Part model, mm, in its own coordinate system. A direction names the side the tool comes from. Coordinates: 2 decimals unless noted, no trailing zeros. Order: outer loops, then holes, each group sorted by start corner. A loop starts at its lowest first (then second) coordinate and runs counter-clockwise, first axis right, second up.
1) Cut at C-C (z = -1.85). List the corners of the cut face in (x, y) (3 decimals).
2) Cut at B-B (y = 18). List the corners of the cut face in (x, z).
3) Wall check: L1, parallel to Y at x = 11, z = -2.2; L2, parallel to X at y = 13.25, z = -1.5; L3, parallel to Y at x = 5, z = -0.8 (3 decimals). Give the ranges that are in metal, low to high.
4) Cut at A-A (x = 5). List the corners of the cut face in (y, z) (3 decimals), and give its area (3 significant figures).
5) Mould opens along Y. For faces 6 (the cylindrical face through (14, 27, -1)), 7 (the cylindrical face through (11, 28, -1)), 8 (the cylindrical face through (8.6, 23.43, -1.48)), 9 (the flat face through (-10, 19, -3)) say: +Y half, -Y half, draft (parallel to the pull), parting line (faces both ways), or undercut.
6) Pin check, flat tips, straight feed: pin 1 Ø0.9 at (y, z) = (1, -1.5) entering from -X; pin 2 Ø1.5 at (y, z) = (17, -1) entering from +X; pin 3 Ø1.1 at (x, z) = (10.5, -1.5) entering from -Y. Stop position of each tip, or through.
7) Cut at D-D (x = -12). List the corners of the cut face in (y, z).
8) Tool access for faces 1 (the cylindrical face through (-19.85, 22.66, -1.48)), 2 (the flat face through (-32, 2.976, -1)), 3 (the flat face through (8, 14, -1)), 4 (the flat face through (-10, 19, 0)), 5 (the cylindrical face through (1.434, 20.389, -1.479)): list every direction of +Z, -Z, +X, -X, +Y, -Y with a clear straight run to the whole face (end or side of a thin tool).
Autodesk Inventor part; units mm, degrees
ref_plane "YZ Plane" through (0, 0, 0) normal (1, 0, 0) x (0, 1, 0)
ref_plane "XZ Plane" through (0, 0, 0) normal (0, 1, 0) x (-1, 0, 0)
ref_plane "XY Plane" through (0, 0, 0) normal (0, 0, 1) x (1, 0, 0)
sketch "Sketch1" plane through (0, 0, 0) normal (0, 0, 1) x (1, 0, 0)
  arc A0 (0, 18) -> (-18, 0.0024) centre (0, 0) ccw
  line L0 (0, 0) -> (0, -6.19)
  line L1 (0, -6.19) -> (2, -6.19)
  arc A1 (2, 30) -> (-33.6563, 0.0024) centre (2, -6.19) ccw
  line L2 (-33.6563, 0.0024) -> (-18, 0.0024)
  line L3 (3, 0) -> (3, 0)
  line L4 (6, 0) -> (32.7783, 0) construction
  line L5 (-33.6563, 0.0024) -> (-33.6563, 30.0024)
  line L6 (2, 30) -> (11, 30)
  line L7 (2, 30) -> (11, 30) construction
  line L8 (0, 0) -> (0, 3)
  line L9 (3, 3) -> (3, 3)
  line L10 (0, 3) -> (2, 3)
  line L11 (2, 6) -> (2, 16)
  line L12 (5, 3) -> (5, 3)
  line L13 (8, 6) -> (8, 22)
  arc A2 (2, 6) -> (5, 3) centre (5, 6) ccw
  arc A3 (5, 3) -> (8, 6) centre (5, 6) ccw
  arc A4 (2, 16) -> (0, 18) centre (0, 16) ccw
  arc A5 (11, 24) -> (11, 30) centre (11, 27) ccw
  line L14 (11, 24) -> (10, 24)
  arc A6 (10, 24) -> (8, 22) centre (10, 22) ccw
  circle A7 centre (5, 6) radius 1
  circle A8 centre (11, 27) radius 1
  line L15 (-33.6563, 0.0024) -> (-31.6563, 0.0024)
  line L16 (-27.1563, 0.0024) -> (-25.1563, 0.0024)
  point P0 (8, 3)
  point P1 (8, 24)
  point P2 (2, 17.8885)
  point P3 (-20.6563, 0.0024)
  dimension "d0" = 36
  dimension "d1" = 6.19
  dimension "d2" = 2
  dimension "d3" = 72.38
  dimension "d11" = 30
  dimension "d14" = 3
  dimension "d17" = 2
  dimension "d18" = 6
  dimension "d19" = 3
  dimension "d20" = 2
  dimension "d21" = 9
  dimension "d23" = 6
  dimension "d24" = 18
  dimension "d25" = 2
  dimension "d26" = 2
  dimension "d27" = 2
  dimension "d28" = 2
  dimension "d31" = 2
extrude "Extrusion1" add sketch "Sketch1" against normal blind 3
sketch "Sketch2" plane through (0, 0, 0) normal (0, 0, 1) x (1, 0, 0)
  arc A0 (0.0129, 20.9952) -> (-17.9376, 1.4977) centre (-0.0001, 2.9953) ccw
  arc A1 (2, 18.9952) -> (-0.013, 20.9952) centre (-0.0001, 18.9952) ccw
  line L0 (2, 18.9952) -> (2, 16.0083)
  circle A2 centre (5, 6.9952) radius 3
  circle A3 centre (5, 6.9952) radius 1
  line L1 (8, 6) -> (8, 22)
  line L2 (-33, 2.9952) -> (-18, 2.9952)
  line L3 (-20, -0.0048) -> (-20, 2.9952)
  line L4 (-24.5, -0.0048) -> (-20, -0.0048)
  line L5 (-24.5, 2.9952) -> (-24.5, -0.0048)
  line L6 (-26.5, -0.0048) -> (-26.5, 2.9952)
  line L7 (-31, -0.0048) -> (-26.5, -0.0048)
  line L8 (-33.6563, 0.0024) -> (-18, 0.0024)
  arc A4 (0, 18) -> (-17.9376, 1.4977) centre (0, 0) ccw
  arc A5 (2, 16) -> (0, 18) centre (0, 16) ccw
  line L9 (2, 16) -> (2, 6)
  arc A6 (2, 6) -> (8, 6) centre (5, 6) ccw
  line L10 (8, 6) -> (8, 22)
  arc A7 (8, 22) -> (10, 24) centre (10, 22) ccw
  line L11 (10, 24) -> (11, 24)
  arc A8 (11, 24) -> (11, 30) centre (11, 27) ccw
  line L12 (11, 30) -> (2, 30)
  arc A9 (2, 30) -> (-33.6563, 0.0024) centre (2, -6.19) ccw
  circle A10 centre (11, 27) radius 1
  circle A11 centre (5, 6) radius 1
  line L13 (-31, 2.9952) -> (-31, -0.0048)
extrude "Extrusion2" cut sketch "Sketch2" against normal blind 9.35 contours A1 L0 A5 A4 A0
sketch "Sketch4" plane through (0, 0, 0) normal (0, 0, 1) x (1, 0, 0)
  circle A0 centre (5, 6) radius 1
  point P0 (0, 0)
extrude "Extrusion3" add sketch "Sketch4" against normal blind 3
sketch "Sketch5" plane through (0, 0, 0) normal (0, 0, 1) x (1, 0, 0)
  line L0 (5, 6) -> (5, 6.995) construction
  circle A0 centre (5, 6.995) radius 1
  point P0 (0, 0)
  dimension "d40" = 0.995
  dimension "d41" = 2
extrude "Extrusion4" cut sketch "Sketch5" against normal blind 3
sketch "Sketch6" plane through (0, 0, 0) normal (0, 0, 1) x (1, 0, 0)
  arc A0 (2, 6) -> (8, 6) centre (5, 6) ccw
  line L0 (5, 6) -> (5, 7)
  circle A1 centre (5, 7) radius 3
  line L1 (2, 16) -> (2, 6)
  line L2 (8, 6) -> (8, 22)
  point P0 (0, 0)
  point P1 (8, 7)
  point P2 (2, 7)
  dimension "d44" = 1
  dimension "d45" = 6
extrude "Extrusion5" cut sketch "Sketch6" against normal blind 3 contours L1 A1 L2 A0
sketch "Sketch8" plane through (0, 0, 0) normal (0, 0, 1) x (1, 0, 0)
  arc A0 (2, 30) -> (-33.6563, 0.0024) centre (2, -6.19) ccw
  line L0 (-33.01, 2.9759) -> (-31.01, 2.9759)
  line L1 (-31.01, 2.9759) -> (-31.01, -0.0241)
  line L2 (-31.01, -0.0241) -> (-26.5101, 0.0024)
  line L3 (-18, 0.0024) -> (-33.6563, 0.0024)
  line L4 (-26.5101, 0.0024) -> (-26.5278, 3.0024)
  line L5 (-26.5278, 3.0024) -> (-24.5279, 2.9759)
  line L6 (-24.5279, 2.9759) -> (-24.4163, -0.022)
  line L7 (-24.4163, -0.022) -> (-19.9163, 0.0024)
  line L8 (-19.9163, 0.0024) -> (-19.9326, 3.0024)
  line L9 (-19.9326, 3.0024) -> (-17.9328, 2.9759)
  arc A1 (2, 30) -> (-33.6563, 0.0024) centre (2, -6.19) ccw
  circle A2 centre (11, 27) radius 1
  arc A3 (2, 7) -> (8, 7) centre (5, 7) ccw
  line L10 (8, 7) -> (8, 22)
  arc A4 (10, 24) -> (8, 22) centre (10, 22) ccw
  line L11 (10, 24) -> (11, 24)
  arc A5 (11, 24) -> (11, 30) centre (11, 27) ccw
  line L12 (11, 30) -> (2, 30)
  arc A6 (2, 30) -> (-33.6563, 0.0024) centre (2, -6.19) ccw
  line L13 (-33.6563, 0.0024) -> (-18, 0.0024)
  arc A7 (-17.9376, 1.4977) -> (-18, 0.0024) centre (0, 0) ccw
  arc A8 (0.0129, 20.9952) -> (-17.9376, 1.4977) centre (-0.0001, 2.9953) ccw
  arc A9 (2, 18.9952) -> (0.0129, 20.9952) centre (-0.0001, 18.9952) ccw
  line L14 (2, 18.9952) -> (2, 16.0083)
  arc A10 (2, 16) -> (2, 16.0083) centre (0, 16) ccw
  line L15 (2, 16) -> (2, 7)
  circle A11 centre (5, 6.995) radius 1
  point P0 (-18, 2.9768)
  point P1 (-31.01, 0.0024)
  point P2 (-24.4172, 0.0024)
  dimension "d48" = 2
  dimension "d49" = 3
  dimension "d50" = 4.5
  dimension "d51" = 3
  dimension "d52" = 2
  dimension "d53" = 3
  dimension "d54" = 4.5
  dimension "d55" = 3
  dimension "d56" = 2
extrude "Extrusion6" cut sketch "Sketch8" against normal blind 3 contours L0 L1 L3 A0 | L4 L5 L6 L3 | L8 L9 A8 A7 L3
properties part number "hinge"
Geometry check:
1. outline: (-33.01, 2.976) - (-31.01, 2.976) - (-31.01, 0.002) - (-26.51, 0.002) - (-26.528, 3.002) - (-24.528, 2.976) - (-24.417, 0.002) - (-19.916, 0.002) - (-19.933, 3.002) - (-18, 2.977) arc R18 cw to (0.013, 20.995) arc R2 cw to (2, 18.995) - (2, 16.008) arc R2 cw to (2, 16) - (2, 7) arc R3 ccw to (8, 7) - (8, 22) arc R2 cw to (10, 24) - (11, 24) arc R3 ccw to (11, 30) - (2, 30) arc R36.19 ccw to start; hole circle Ø2 at (5, 6.995); hole circle Ø2 at (11, 27)
2. outline: (-24.92, -3) - (-9.94, -3) - (-9.94, 0) - (-24.92, 0) - close; (2, -3) - (8, -3) - (8, 0) - (2, 0) - close
3. L1: y = 24 to 26, 28 to 30
3. L2: x = -28.53 to -14.79, 2 to 8
3. L3: y = 4 to 5.995, 7.995 to 30
4. outline: (4, -3) - (5.995, -3) - (5.995, 0) - (4, 0) - close; (7.995, -3) - (30, -3) - (30, 0) - (7.995, 0) - close
4. area: 72.0 mm2
5. face 6: parting line
5. face 7: undercut
5. face 8: -Y half
5. face 9: draft
6. pin 1: stops at x = -31.01
6. pin 2: stops at x = 8
6. pin 3: stops at y = 24
7. outline: (16.41, -3) - (27.18, -3) - (27.18, 0) - (16.41, 0) - close
8. face 1: +Z, -Z, -X, +Y
8. face 2: +Z, -Z, -X, -Y
8. face 3: +Z, -Z, +X, -Y
8. face 4: +Z, +X, -X, +Y, -Y
8. face 5: +Z, -Z, -Y
